Check sheet for the modelled part. Datum: model origin and axes. Units: mm. Face numbers are marked on the shaded views. A direction names the side the tool comes from. Give positions to 0.01 mm unless a question says otherwise; leave off trailing zeros. Write each loop counter-clockwise with the first axis right and the second up, starting at its lowest first coordinate (ties: lowest second). Pieces come first, ordered by that corner, then holes. Notation, with made-up numbers: M -17.5,79.5 L 30.5,79.5 A20 ccw 30.5,93.5 Z; hole C 81,36 d1. An arc over 180 degrees is marked long. One line per item, written item: value. Start each with the question number.
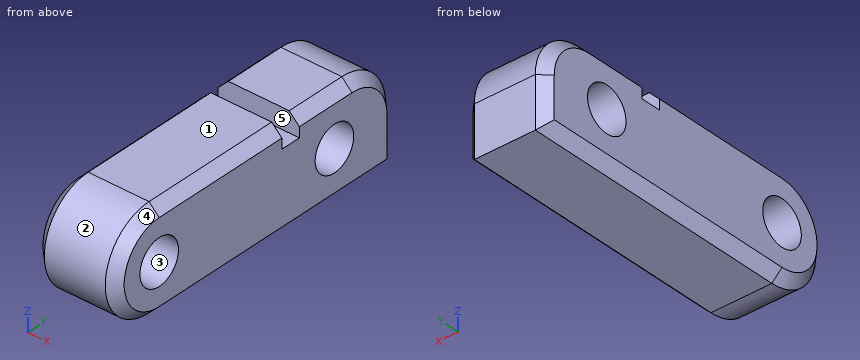
Autodesk Inventor part; units mm, degrees
ref_plane "YZ Plane" through (0, 0, 0) normal (1, 0, 0) x (0, 1, 0)
ref_plane "XZ Plane" through (0, 0, 0) normal (0, 1, 0) x (-1, 0, 0)
ref_plane "XY Plane" through (0, 0, 0) normal (0, 0, 1) x (1, 0, 0)
sketch "Skizze1" plane through (0, 0, 0) normal (1, 0, 0) x (0, 1, 0)
  line L0 (0, 0) -> (-10, 0) construction
  circle A0 centre (0, 0) radius 1.1
  circle A1 centre (-10, 0) radius 1.1
  arc A2 (-10, 2.5) -> (-10, -2.5) centre (-10, 0) ccw
  line L1 (-10, -2.5) -> (3.5, -2.5)
  line L2 (-10, 2.5) -> (1, 2.5)
  arc A3 (3.5, 0) -> (1, 2.5) centre (1, 0) ccw
  line L3 (3.5, 0) -> (3.5, -2.5)
  dimension "d0" = 10
  dimension "d1" = 2.2
  dimension "d2" = 2.2
  dimension "d3" = 2.5
  dimension "d8" = 2.5
  dimension "d9" = 3.5
extrude "Extrusion1" add sketch "Skizze1" along normal mid plane 4
chamfer "Fase1" distance 0.5 angle 45 10 edges at (2, 2.7678, 1.7678) (2, -4.5, 2.5) (2, -12.5, 0) (2, -3.25, -2.5) (2, 3.5, -1.25) (-2, 2.7678, 1.7678) (-2, -4.5, 2.5) (-2, -12.5, 0) (-2, -3.25, -2.5) (-2, 3.5, -1.25)
sketch "Skizze5" plane through (-1.5, -10, 2.5) normal (0, 0, 1) x (1, 0, 0)
  line L0 (1.5, 16.7) -> (1.5, -5.7)
  line L1 (-1.3, 10) -> (4.3, 10)
  line L2 (3.5, 8) -> (-0.5, 8)
  line L3 (-0.5, 8) -> (-0.5, 7)
  line L4 (-0.5, 7) -> (3.5, 7)
  line L5 (3.5, 7) -> (3.5, 8)
  line L6 (3.5, 0) -> (3.5, 11)
  line L7 (-0.5, 11) -> (-0.5, 0)
  point P0 (1.5, 10)
  dimension "d26" = 1
  dimension "d27" = 2
extrude "Extrusion4" cut sketch "Skizze5" against normal blind 1 contours L2 L5 L4 L0 | L0 L4 L3 L2
pattern_linear "Rechteckige Anordnung1" [suppressed]
equation "\"d2\" = d1"
properties part number "Chipanschlag TN2"
1) Gauge pin test, flat ends, axial feed: pin 1 (2 mm diameter, centred on x = 0.5, z = -1.5, fed in from -Y); pin 2 (0.8 mm diameter, centred on x = 0.5, z = 2, fed in from +Y); pin 3 (0.5 mm diameter, centred on x = 0, z = 2, fed in from -Y). Record the tip position at first contact, or that the pin passes through.
2) Tool access check on the marked faces 4 and 5. Record the directions out of +Z, -Z, +X, -X, +Y, -Y that give a thin tool (end or side, any length) a straight path to the whole face; none if there is none.
3) Cross-section at B-B (y = 0). Record the boundary of the cut face in (x, z), plus the area to 3 significant figures.
4) Cross-section at C-C (y = -2.25). Record the boundary of the cut face in (x, z), plus the area to 4 significant figures.
5) Cross-section at A-A (x = -0.35). Record the boundary of the cut face in (y, z).
6) Cross-section at D-D (z = 0.4). State how many separate pieces and enclosed holes the cut face has, plus the area to 3 significant figures.
7) Material ranges on L1, parallel to Z at x = -0.95, y = -10; L2, parallel to Y at x = -1.75, z = 0.45; L3, parallel to Y at x = -0.1, z = 0.7, recorded low to high. Write a range as from..to.
8) Draft check along Z on the marked faces 1, 2 and 3. Enter one of: released by +Z, released by -Z, zero draft, split by the parting line, or undercut.
Data:
1. pin 1: stops at y = -12.45
1. pin 2: stops at y = 2.92
1. pin 3: stops at y = -11.79
2. face 4: +X, -Y
2. face 5: +Z, +X, -X
3. outline: M -2,-2 L -1.5,-2.5 L 1.5,-2.5 L 2,-2 L 2,-1.1 L -2,-1.1 Z; M -2,1.1 L 2,1.1 L 2,2 L 1.5,2.5 L -1.5,2.5 L -2,2 Z
3. area: 10.7 mm2
4. outline: M -2,-2 L -1.5,-2.5 L 1.5,-2.5 L 2,-2 L 2,1.5 L -2,1.5 Z
4. area: 15.75 mm2
5. outline: M -10,-2.5 L 3.5,-2.5 L 3.5,0 A2.5 ccw 1,2.5 L -2,2.5 L -2,1.5 L -3,1.5 L -3,2.5 L -10,2.5 A2.5 ccw Z; hole C -10,0 d2.2; hole C 0,0 d2.2
6. separate pieces: 3
6. enclosed holes: 0
6. area: 46.8 mm2
7. L1: z = -2.5..-1.1, 1.1..2.5
7. L2: y = -12.2..-11, -9..-1, 1..3.2
7. L3: y = -12.4..-10.85, -9.15..-0.85, 0.85..3.4
8. face 1: released by +Z
8. face 2: split by the parting line
8. face 3: undercut
